Input: part model. Units: mm. Frame: model coordinates. Face numbers are marked on the shaded views. Coordinates: 2 decimals unless noted, no trailing zeros. Loops run counter-clockwise (first coordinate to the right, second up) from the corner with the lowest first, then second, coordinate; pieces in that order, holes last. Notation, with made-up numbers: M -34,-10 L -1,-10 A19 ccw -1,2 Z; hole C 33,-31 d4. An arc over 180 degrees is marked long. Use a Markdown table: item, result. Add a question column.
1. Pin query (flat end, axial travel): pin 1 (1 mm diameter, centred on y = 4, z = 2.5, fed in from -X); pin 2 (1.5 mm diameter, centred on y = 1, z = -1, fed in from +X); pin 3 (1.5 mm diameter, centred on x = -3.5, y = 3.5, fed in from +Z). Return the tip coordinate at first contact, or that it passes through.
2. Section A-A on y = 1.55. Output: boundary loops of the cut face in (x, z).
3. Draft query along Z for the marked faces 1, 2, 3 and 4. Return one class per face: +Z half, -Z half, draft (parallel to the pull), parting line (faces both ways), or undercut.
4. Line query: L1, parallel to Z at x = 1, y = 1.25; L2, parallel to X at y = 1.05, z = -1.5; L3, parallel to Z at x = -0.25, y = 4.1. Output: solid intervals per line, ascending. Write a range as [from, to].
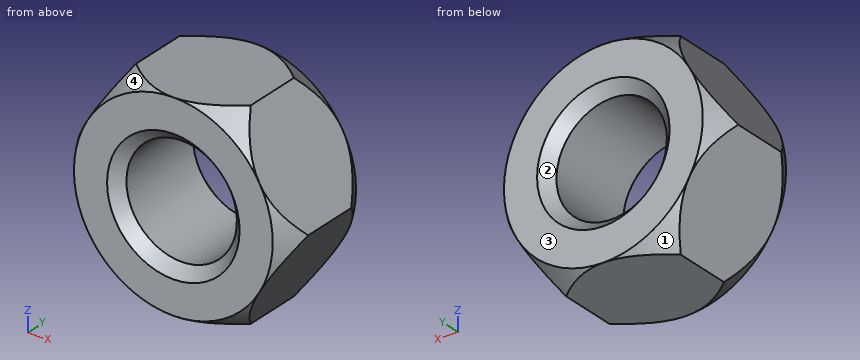
```python
from build123d import *

# Parameters (mm, degrees)
EXTRUDE_1_DEPTH     = 5
SKETCH_2_R          = 2.5
CUT_EXTRUDE_1_DEPTH = 5
SKETCH_3_OUTSIDE_W  = 21.092
SKETCH_3_OUTSIDE_H  = 19.7
SKETCH_3_OUTSIDE_R  = 4.5
CUT_EXTRUDE_2_DEPTH = 5
CUT_EXTRUDE_2_DRAFT = -30
SKETCH_4_OUTSIDE_W  = 21.092
SKETCH_4_OUTSIDE_H  = 19.7
SKETCH_4_OUTSIDE_R  = 4.5
CUT_EXTRUDE_3_DEPTH = 5
CUT_EXTRUDE_3_DRAFT = -30
CHAMFER_1_SIZE      = 0.5
CHAMFER_2_SIZE      = 0.5


with BuildPart() as part:
    # 草图1 → 凸台-拉伸1 (new body)
    with BuildSketch(Plane(origin=(0, 0, 0), x_dir=(1, 0, 0), z_dir=(0, 1, 0))):
        Polygon((2.598076211, 4.5), (-2.598076211, 4.5), (-5.196152423, 0), (-2.598076211, -4.5), (2.598076211, -4.5), (5.196152423, 0), align=None)
    extrude(amount=EXTRUDE_1_DEPTH)

    # 草图2 → 切除-拉伸1 (cut)
    with BuildSketch(Plane(origin=(0, 5, 0), x_dir=(1, 0, 0), z_dir=(0, 1, 0))):
        with Locations(Location((0, 0, 0), (0, 0, 270))):
            Circle(SKETCH_2_R)
    extrude(amount=-CUT_EXTRUDE_1_DEPTH, mode=Mode.SUBTRACT)


with BuildPart() as cut_extrude_2_tool:
    # 草图3 outside → 切除-拉伸2 (with draft: the straight prism first)
    with BuildSketch(Plane(origin=(0, 5, 0), x_dir=(1, 0, 0), z_dir=(0, 1, 0))):
        Rectangle(SKETCH_3_OUTSIDE_W, SKETCH_3_OUTSIDE_H)
        Circle(SKETCH_3_OUTSIDE_R, mode=Mode.SUBTRACT)
    extrude(amount=-CUT_EXTRUDE_2_DEPTH)
    # 切除-拉伸2: the draft: its side faces are tilted about the plane it starts from
    cut_extrude_2_sides = [cut_extrude_2_tool.faces().sort_by_distance(p)[0] for p in [
        (0, 2.5, 9.85),
        (10.546, 2.5, 0),
        (0, 2.5, -9.85),
        (-10.546, 2.5, 0),
        (-4.5, 2.5, 0),
    ]]
    draft(cut_extrude_2_sides, Plane(origin=(0, 5, 0), x_dir=(1, 0, 0), z_dir=(0, 1, 0)), CUT_EXTRUDE_2_DRAFT)


with BuildPart() as part_1:
    add(part.part)

    # 切除-拉伸2: cut by cut_extrude_2_tool
    add(cut_extrude_2_tool.part, mode=Mode.SUBTRACT)


with BuildPart() as cut_extrude_3_tool:
    # 草图4 outside → 切除-拉伸3 (with draft: the straight prism first)
    with BuildSketch(Plane.XZ):
        Rectangle(SKETCH_4_OUTSIDE_W, SKETCH_4_OUTSIDE_H)
        Circle(SKETCH_4_OUTSIDE_R, mode=Mode.SUBTRACT)
    extrude(amount=-CUT_EXTRUDE_3_DEPTH)
    # 切除-拉伸3: the draft: its side faces are tilted about the plane it starts from
    cut_extrude_3_sides = [cut_extrude_3_tool.faces().sort_by_distance(p)[0] for p in [
        (0, 2.5, -9.85),
        (10.546, 2.5, 0),
        (0, 2.5, 9.85),
        (-10.546, 2.5, 0),
        (-4.5, 2.5, 0),
    ]]
    draft(cut_extrude_3_sides, Plane.XZ, CUT_EXTRUDE_3_DRAFT)


with BuildPart() as part_2:
    add(part_1.part)

    # 切除-拉伸3: cut by cut_extrude_3_tool
    add(cut_extrude_3_tool.part, mode=Mode.SUBTRACT)

    # 倒角1
    chamfer_1_edges = [part_2.edges().sort_by_distance(p)[0] for p in [
        (0, 5, -2.5),
    ]]
    chamfer(chamfer_1_edges, length=CHAMFER_1_SIZE)

    # 倒角2
    chamfer_2_edges = [part_2.edges().sort_by_distance(p)[0] for p in [
        (0, 0, -2.5),
    ]]
    chamfer(chamfer_2_edges, length=CHAMFER_2_SIZE)


solid = part_2.part
```
Answers below:
| question | item | result |
|---|---|---|
| 1 | pin 1 | stops at x = -4.04 |
| 1 | pin 2 | stops at x = 5.05 |
| 1 | pin 3 | stops at z = 4.24 |
| 2 | outline | M -5.2,0 L -2.6,-4.5 L 2.6,-4.5 L 5.2,0 L 2.6,4.5 L -2.6,4.5 Z; hole C 0,0 d5 |
| 3 | face 1 | -Z half |
| 3 | face 2 | undercut |
| 3 | face 3 | draft |
| 3 | face 4 | +Z half |
| 4 | L1 | z = [-4.5, -2.29], [2.29, 4.5] |
| 4 | L2 | x = [-4.33, -2], [2, 4.33] |
| 4 | L3 | z = [-4.5, -2.49], [2.49, 4.5] |
